from build123d import *

# Parameters (mm, degrees)
SKETCH13_W          = 15
SKETCH13_H          = 15
BOSS_EXTRUDE3_DEPTH = 420
BOSS_EXTRUDE4_START = -70
SKETCH12_W          = 15
SKETCH12_H          = 15
BOSS_EXTRUDE4_DEPTH = 110
SKETCH14_W          = 5
SKETCH14_H          = 5
BOSS_EXTRUDE5_DEPTH = 6
FILLET1_R           = 2
FILLET2_R           = 1
FILLET3_R           = 2
FILLET4_R           = 2
SKETCH15_R          = 3
CUT_EXTRUDE1_DEPTH  = 402.04987221


with BuildPart() as part:
    # Sketch13 → Boss-Extrude3 (new body)
    with BuildSketch(Plane.XY.offset(-50)):
        with Locations((0, 45.5)):
            Rectangle(SKETCH13_W, SKETCH13_H)
    extrude(amount=BOSS_EXTRUDE3_DEPTH)

    # Sketch12 → Boss-Extrude4 (add)
    with BuildSketch(Plane(origin=(0, 108, 0), x_dir=(1, 0, 0), z_dir=(0, 1, 0)).offset(BOSS_EXTRUDE4_START)):
        with Locations((0, 7.5)):
            Rectangle(SKETCH12_W, SKETCH12_H)
    extrude(amount=BOSS_EXTRUDE4_DEPTH)

    # Sketch14 → Boss-Extrude5 (add)
    with BuildSketch(Plane(origin=(0, 148, 0), x_dir=(1, 0, 0), z_dir=(0, 1, 0))):
        with Locations((0, 7.5)):
            Rectangle(SKETCH14_W, SKETCH14_H)
    extrude(amount=BOSS_EXTRUDE5_DEPTH)

    # Fillet1
    fillet1_edges = [part.edges().sort_by_distance(p)[0] for p in [
        (-7.5, 45.5, 370),
        (0, 38, 370),
        (-7.5, 53, -32.5),
        (7.5, 53, -32.5),
        (-7.5, 100.5, -15),
        (-7.5, 100.5, 0),
        (0, 53, 0),
        (7.5, 100.5, 0),
        (7.5, 100.5, -15),
        (0, 53, -15),
        (-7.5, 148, -7.5),
        (0, 148, 0),
        (7.5, 148, -7.5),
        (0, 148, -15),
        (0, 38, -50),
        (-7.5, 45.5, -50),
        (7.5, 45.5, -50),
        (7.5, 38, 160),
        (-7.5, 38, 160),
        (-7.5, 53, 185),
        (7.5, 53, 185),
        (0, 53, 370),
    ]]
    fillet(fillet1_edges, radius=FILLET1_R)

    # Fillet2
    fillet2_edges = [part.edges().sort_by_distance(p)[0] for p in [
        (2.5, 148, -7.5),
        (0, 148, -10),
        (-2.5, 148, -7.5),
        (0, 148, -5),
        (2.5, 154, -7.5),
        (0, 154, -10),
        (-2.5, 154, -7.5),
        (0, 154, -5),
    ]]
    fillet(fillet2_edges, radius=FILLET2_R)

    # Fillet3
    # the kernel refuses this fillet: 2 mm, written as the material it takes off along each edge
    with BuildSketch(Plane(origin=(5.5, 51, 368), x_dir=(0, 0, 1), z_dir=(1, 0, 0))) as fillet3_piece_1_section:
        Polygon((0, 0), (FILLET3_R, 0), (FILLET3_R, -FILLET3_R), (0, -FILLET3_R), align=None)
    fillet3_piece_1 = extrude(amount=FILLET3_R, mode=Mode.PRIVATE)
    fillet3_piece_1 = fillet3_piece_1 - Plane(origin=(5.5, 51, 368), x_dir=(0, -0.7071067811865475, -0.7071067811865475), z_dir=(1, 0, 0)) * Sphere(FILLET3_R, mode=Mode.PRIVATE)
    add(fillet3_piece_1, mode=Mode.SUBTRACT)
    with BuildSketch(Plane(origin=(5.5, 40, 368), x_dir=(0, 0, 1), z_dir=(1, 0, 0))) as fillet3_piece_2_section:
        Polygon((0, 0), (FILLET3_R, 0), (FILLET3_R, FILLET3_R), (0, FILLET3_R), align=None)
    fillet3_piece_2 = extrude(amount=FILLET3_R, mode=Mode.PRIVATE)
    fillet3_piece_2 = fillet3_piece_2 - Plane(origin=(5.5, 40, 368), x_dir=(0, 0.7071067811865475, -0.7071067811865475), z_dir=(1, 0, 0)) * Sphere(FILLET3_R, mode=Mode.PRIVATE)
    add(fillet3_piece_2, mode=Mode.SUBTRACT)
    with BuildSketch(Plane(origin=(7.5, 51, 370), x_dir=(0, 0, -1), z_dir=(0, -1, 0))) as fillet3_piece_3:
        with BuildLine():
            CenterArc((FILLET3_R, -FILLET3_R), FILLET3_R, 90, 90)
            Line((0, -FILLET3_R), (0, 0))
            Line((0, 0), (FILLET3_R, 0))
        make_face()
    extrude(amount=11, mode=Mode.SUBTRACT)

    # Fillet4
    # the kernel refuses this fillet: 2 mm, written as the material it takes off along each edge
    with BuildSketch(Plane(origin=(-5.5, 51, -48), x_dir=(0, 1, 0), z_dir=(0, 0, -1))) as fillet4_piece_1_section:
        Polygon((0, 0), (FILLET4_R, 0), (FILLET4_R, -FILLET4_R), (0, -FILLET4_R), align=None)
    fillet4_piece_1 = extrude(amount=FILLET4_R, mode=Mode.PRIVATE)
    fillet4_piece_1 = fillet4_piece_1 - Plane(origin=(-5.5, 51, -48), x_dir=(0.7071067811865472, -0.7071067811865478, 0), z_dir=(0, 0, -1)) * Sphere(FILLET4_R, mode=Mode.PRIVATE)
    add(fillet4_piece_1, mode=Mode.SUBTRACT)
    with BuildSketch(Plane(origin=(5.5, 51, -48), x_dir=(0, 1, 0), z_dir=(0, 0, -1))) as fillet4_piece_2_section:
        Polygon((0, 0), (FILLET4_R, 0), (FILLET4_R, FILLET4_R), (0, FILLET4_R), align=None)
    fillet4_piece_2 = extrude(amount=FILLET4_R, mode=Mode.PRIVATE)
    fillet4_piece_2 = fillet4_piece_2 - Plane(origin=(5.5, 51, -48), x_dir=(-0.7071067811865479, -0.7071067811865472, 0), z_dir=(0, 0, -1)) * Sphere(FILLET4_R, mode=Mode.PRIVATE)
    add(fillet4_piece_2, mode=Mode.SUBTRACT)
    with BuildSketch(Plane(origin=(-5.5, 53, -50), x_dir=(0, -1, 0), z_dir=(1, 0, 0))) as fillet4_piece_3:
        with BuildLine():
            CenterArc((FILLET4_R, -FILLET4_R), FILLET4_R, 90, 90)
            Line((0, -FILLET4_R), (0, 0))
            Line((0, 0), (FILLET4_R, 0))
        make_face()
    extrude(amount=11, mode=Mode.SUBTRACT)

    # Sketch15 → Cut-Extrude1 (cut, through all)
    with BuildSketch(Plane.ZY.offset(7.5)):
        with Locations(Location((15, 45.5, 0), (0, 0, 270))):
            Circle(SKETCH15_R)
    extrude(amount=-CUT_EXTRUDE1_DEPTH, mode=Mode.SUBTRACT)


solid = part.part
Input: part model. Units: mm. Frame: model coordinates. A direction names the side the tool comes from. Give positions to 0.01 mm unless a question says otherwise; leave off trailing zeros. Order: outer loops, then holes, each group sorted by start corner. A loop starts at its lowest first (then second) coordinate and runs counter-clockwise, first axis right, second up.
Q1. Section A-A on y = 123. Output: boundary loops of the cut face in (x, z), and give its area (3 significant figures).
Checked values:
outline: (-7.5, -13) arc R2 ccw to (-5.5, -15) - (5.5, -15) arc R2 ccw to (7.5, -13) - (7.5, -2) arc R2 ccw to (5.5, 0) - (-5.5, 0) arc R2 ccw to (-7.5, -2) - close
area: 222 mm2
Q2. Ray query, probe 1 along Z at (x, y) = (1, 45.5); probe 2 along Z at (x, y) = (3.5, 64); probe 3 along Y at (x, z) = (-2, 184). Return the intervals inside material, ascending.
Checked values:
probe 1: z = -50 to 12, 18 to 370
probe 2: z = -15 to 0
probe 3: y = 38 to 53
Q3. Set-up query: faces 1 (the flat face through (-4, 148, -8)), 2 (the flat face through (0, 38, 157)), 3 (the flat face through (0, 100, -15)), 4 (the flat face through (0, 100, 0)). Return all of +Z, -Z, +X, -X, +Y, -Y with unobstructed straight access to the full face (end or side cutting, diameter ignored); none if empty.
Checked values:
face 1: +Y
face 2: +Z, -Z, +X, -X, -Y
face 3: -Z, +X, -X, +Y
face 4: +Z, +X, -X, +Y
Q4. Contact query for flat-ended pins moving along their axis: pin 1 Ø1.2 at (y, z) = (152, -8.5) entering from +X; pin 2 Ø9 at (x, y) = (-1, 117.5) entering from -Z; pin 3 Ø2 at (x, z) = (4, 285) entering from +Y. Output: stop coordinate, or through.
Checked values:
pin 1: stops at x = 2.5
pin 2: stops at z = -15
pin 3: stops at y = 53
Q5. Section B-B on z = 311. Output: boundary loops of the cut face in (x, y).
Checked values:
outline: (-7.5, 40) arc R2 ccw to (-5.5, 38) - (5.5, 38) arc R2 ccw to (7.5, 40) - (7.5, 51) arc R2 ccw to (5.5, 53) - (-5.5, 53) arc R2 ccw to (-7.5, 51) - close
